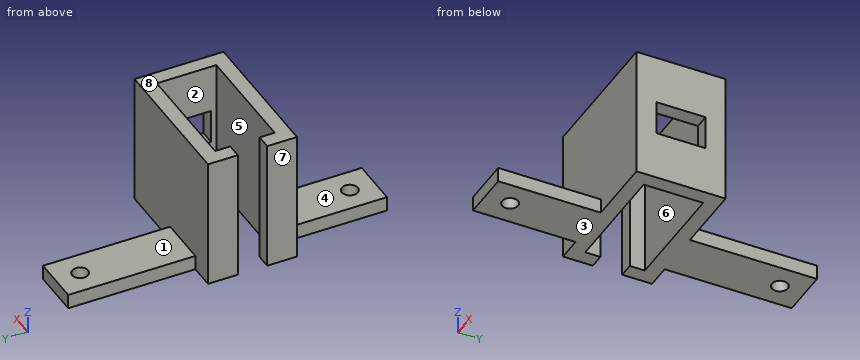
from build123d import *

# Parameters (mm, degrees)
ESQUISSE1_W                = 10
ESQUISSE1_H                = 25.925
BOSS_EXTRU_1_DEPTH         = 3
ESQUISSE1_H_2              = 20.925
BOSS_EXTRU_1_2_DEPTH       = 3
ESQUISSE1_3_W              = 23.15
ESQUISSE1_3_H              = 12.15
BOSS_EXTRU_2_DEPTH         = 27
ESQUISSE3_R                = 1.625
ENL_V_MAT_EXTRU_2_DEPTH    = 4
R_P_TITION_LIN_AIRE1_COUNT = 2
R_P_TITION_LIN_AIRE1_PITCH = 55
ESQUISSE5_W                = 27
ESQUISSE5_H                = 6
ENL_V_MAT_EXTRU_3_DEPTH    = 10
ENL_V_MAT_EXTRU_4_REACH    = 31.15
ESQUISSE6_W                = 7
ESQUISSE6_H                = 10


with BuildPart() as part:
    # Esquisse1 → Boss.-Extru.1 (new body)
    with BuildSketch(Plane.XY):
        with Locations((5, -12.9625)):
            Rectangle(ESQUISSE1_W, ESQUISSE1_H)
    extrude(amount=BOSS_EXTRU_1_DEPTH)



with BuildPart() as body_2:
    # Esquisse1 → Boss.-Extru.1 2 (new body)
    with BuildSketch(Plane.XY):
        with Locations((5, -54.5375)):
            Rectangle(ESQUISSE1_W, ESQUISSE1_H_2)
    extrude(amount=BOSS_EXTRU_1_2_DEPTH)


with BuildPart() as part_1:
    add(part.part)

    add(body_2.part)  # Boss.-Extru.2 merges body 2
    # Esquisse1_3 → Boss.-Extru.2 (add)
    with BuildSketch(Plane.XY):
        Polygon((10, -44.075), (0, -44.075), (-5, -44.075), (-5, -25.925), (0, -25.925), (10, -25.925), (24.15, -25.925), (24.15, -44.075), align=None)
        with Locations((9.575, -35)):
            Rectangle(ESQUISSE1_3_W, ESQUISSE1_3_H, mode=Mode.SUBTRACT)
    extrude(amount=BOSS_EXTRU_2_DEPTH)

    # Esquisse3 → Enl_v. mat.-Extru.2 (cut, through all)
    with BuildSketch(Plane.XY.offset(3)):
        with Locations((5, -5)):
            Circle(ESQUISSE3_R)
    enl_v_mat_extru_2 = extrude(amount=-ENL_V_MAT_EXTRU_2_DEPTH, mode=Mode.SUBTRACT)

    # R_p_tition lin_aire1: Enl_v. mat.-Extru.2 ×2
    with Locations(*[(0, -i * R_P_TITION_LIN_AIRE1_PITCH, 0) for i in range(1, R_P_TITION_LIN_AIRE1_COUNT)]):
        add(enl_v_mat_extru_2, mode=Mode.SUBTRACT)

    # Esquisse5 → Enl_v. mat.-Extru.3 (cut)
    with BuildSketch(Plane.ZY.offset(5)):
        with Locations((13.5, -35)):
            Rectangle(ESQUISSE5_W, ESQUISSE5_H)
    extrude(amount=-ENL_V_MAT_EXTRU_3_DEPTH, mode=Mode.SUBTRACT)

    # Esquisse6 → Enl_v. mat.-Extru.4 (cut, up to next)
    with BuildSketch(Plane(origin=(24.15, 0, 0), x_dir=(0, 0, -1), z_dir=(1, 0, 0)), mode=Mode.PRIVATE) as enl_v_mat_extru_4_sk1:
        with Locations((-13.5, -35)):
            Rectangle(ESQUISSE6_W, ESQUISSE6_H)
    enl_v_mat_extru_4_tool1 = extrude(enl_v_mat_extru_4_sk1.sketch, amount=-ENL_V_MAT_EXTRU_4_REACH, mode=Mode.PRIVATE) & part_1.part
    add(enl_v_mat_extru_4_tool1.solids().sort_by_distance((24.15, -35, 13.5))[0], mode=Mode.SUBTRACT)


solid = part_1.part
Source: CAD feature listing. Evaluate the final solid. Frame: model axes, mm. Face numbers are marked on the shaded views. A direction names the side the tool comes from. Coordinates: 2 decimals unless noted, no trailing zeros. Loops run counter-clockwise (first coordinate to the right, second up) from the corner with the lowest first, then second, coordinate; pieces in that order, holes last. Notation, with made-up numbers: (-26.75, -16.5) -> (28.25, -16.5) arc R5 cw to (28.25, -7.5) -> close; hole circle Ø10 at (34.5, -2). An arc over 180 degrees is marked (long way). Answer in a Markdown table with one row per item. Add a question column.
Q1. Reachability of the marked faces 1, 2, 3 and 4 from +Z, -Z, +X, -X, +Y, -Y: full face, straight path, thin tool, end or side. Return the list, or none.
Q2. Section B-B on y = -60. Return the cut outline in (x, z) (3 decimals).
Q3. Section D-D on x = 5. Return the cut outline in (y, z) (3 decimals).
Q4. Section A-A on x = 1.5. Return the cut outline in (y, z) (3 decimals).
Q5. Ray query, line 1 along Y through (x, z) = (5, 1.9) (3 decimals); line 2 along Y through (x, z) = (14, 13) (3 decimals); line 3 along Z through (x, y) = (8.25, -23). Return the intervals inside material, ascending.
Q6. Section C-C on z = 2. Return the cut outline in (x, y) (3 decimals), and give its area (3 significant figures).
Q7. Contact query for flat-ended pins moving along their axis: pin 1 Ø4 at (x, z) = (7.5, 6.5) entering from +Y (3 decimals); pin 2 Ø4 at (x, z) = (9, 6) entering from -Y (3 decimals); pin 3 Ø4 at (x, y) = (5, -60) entering from -Z; pin 4 Ø6 at (x, y) = (4.5, -13) entering from +Z. Output: stop coordinate, or through.
Q8. Pull-direction query (X, two-part tool) for the marked faces 5, 6, 7 and 8; classes: pulls with the +X half, pulls with the -X half, needs draft (parallel to the pull), parting line crosses it, or undercut.
Computed values:
| question | item | result |
|---|---|---|
| 1 | face 1 | +Z, +X, -X, +Y |
| 1 | face 2 | +Z, -Z |
| 1 | face 3 | -Z, +X, -X, +Y, -Y |
| 1 | face 4 | +Z, +X, -X, -Y |
| 2 | outline | (0, 0) -> (3.375, 0) -> (3.375, 3) -> (0, 3) -> close; (6.625, 0) -> (10, 0) -> (10, 3) -> (6.625, 3) -> close |
| 3 | outline | (-65, 0) -> (-61.625, 0) -> (-61.625, 3) -> (-65, 3) -> close; (-58.375, 0) -> (-41.075, 0) -> (-41.075, 27) -> (-44.075, 27) -> (-44.075, 3) -> (-58.375, 3) -> close; (-28.925, 0) -> (-6.625, 0) -> (-6.625, 3) -> (-25.925, 3) -> (-25.925, 27) -> (-28.925, 27) -> close; (-3.375, 0) -> (0, 0) -> (0, 3) -> (-3.375, 3) -> close |
| 4 | outline | (-65, 0) -> (-41.075, 0) -> (-41.075, 27) -> (-44.075, 27) -> (-44.075, 3) -> (-65, 3) -> close; (-28.925, 0) -> (0, 0) -> (0, 3) -> (-25.925, 3) -> (-25.925, 27) -> (-28.925, 27) -> close |
| 5 | line 1 | y = -65 to -61.625, -58.375 to -41.075, -28.925 to -6.625, -3.375 to 0 |
| 5 | line 2 | y = -44.075 to -41.075, -28.925 to -25.925 |
| 5 | line 3 | z = 0 to 3 |
| 6 | outline | (-5, -44.075) -> (0, -44.075) -> (0, -65) -> (10, -65) -> (10, -44.075) -> (24.15, -44.075) -> (24.15, -25.925) -> (10, -25.925) -> (10, 0) -> (0, 0) -> (0, -25.925) -> (-5, -25.925) -> (-5, -32) -> (-2, -32) -> (-2, -28.925) -> (21.15, -28.925) -> (21.15, -41.075) -> (-2, -41.075) -> (-2, -38) -> (-5, -38) -> close; hole circle Ø3.25 at (5, -60); hole circle Ø3.25 at (5, -5) |
| 6 | area | 682 mm^2 |
| 7 | pin 1 | stops at y = -25.925 |
| 7 | pin 2 | stops at y = -44.075 |
| 7 | pin 3 | stops at z = 0 |
| 7 | pin 4 | stops at z = 3 |
| 8 | face 5 | undercut |
| 8 | face 6 | undercut |
| 8 | face 7 | pulls with the -X half |
| 8 | face 8 | needs draft |
